from build123d import *

# Parameters (mm, degrees)
F1_DEPTH = 5


with BuildPart() as f1:
    # F0 (on Top) → F1 (new body)
    with BuildSketch(Plane.XY):
        with BuildLine():
            ThreePointArc((1.28e-08, 6), (4.9888176774, 3.3334213928), (5.5432771951, -2.2961005942))
            Line((5.5432771951, -2.2961005942), (5.5432771951, -9.5011619257))
            ThreePointArc((5.5432771951, -9.5011619257), (10.703117819, -2.5383595004), (9.2195444573, 6))
            Line((9.2195444573, 6), (1.28e-08, 6))
        make_face()
        with BuildLine():
            ThreePointArc((-5.5432771951, -2.2961005942), (-4.9888176703, 3.3334214034), (1.28e-08, 6))
            Line((1.28e-08, 6), (-9.2195444573, 6))
            ThreePointArc((-9.2195444573, 6), (-10.703117819, -2.5383595004), (-5.5432771951, -9.5011619257))
            Line((-5.5432771951, -9.5011619257), (-5.5432771951, -2.2961005942))
        make_face()
        with BuildLine():
            Line((-9.2195444573, 6), (1.28e-08, 6))
            Line((1.28e-08, 6), (9.2195444573, 6))
            ThreePointArc((9.2195444573, 6), (5.2440442409, 9.6695398029), (0, 11))
            ThreePointArc((0, 11), (-5.2440442409, 9.6695398029), (-9.2195444573, 6))
        make_face()
        with BuildLine():
            Line((-12, 6), (-9.2195444573, 6))
            ThreePointArc((-9.2195444573, 6), (-5.2440442409, 9.6695398029), (0, 11))
            Line((0, 11), (-12, 11))
            Line((-12, 11), (-12, 6))
        make_face()
        with BuildLine():
            ThreePointArc((0, 11), (5.2440442409, 9.6695398029), (9.2195444573, 6))
            Line((9.2195444573, 6), (12, 6))
            Line((12, 6), (12, 11))
            Line((12, 11), (0, 11))
        make_face()
    extrude(amount=F1_DEPTH)


solid = f1.part
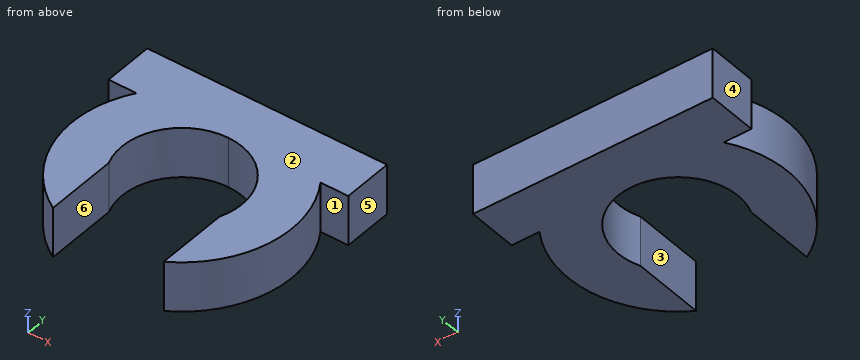
Check sheet for the modelled part. Datum: model origin and axes. Units: mm. Face numbers are marked on the shaded views. A direction names the side the tool comes from. Round coordinates to 2 decimals unless told otherwise and drop trailing zeros. Order: outer loops, then holes, each group sorted by start corner. A loop starts at its lowest first (then second) coordinate and runs counter-clockwise, first axis right, second up.
(1) Cross-section at C-C, the plane x = 9.75. Enter the section's corners in (y, z).
(2) Access from +Z, -Z, +X, -X, +Y, -Y to the whole of each face (thin tool, end or side, straight path). Record for the marked faces 1, 2 and 3.
(3) Cross-section at A-A, the plane y = 0. Enter the section's corners in (x, z).
(4) Draft check along X on the marked faces 4, 5 and 6. Enter one of: pulls with the +X half, pulls with the -X half, needs draft (parallel to the pull), parting line crosses it, or undercut.
(5) Go/stop test with flat-tipped pins: P1, Ø1.5, axis at x = -8, z = 4, coming from the -Y side; P2, Ø2, axis at x = -11, z = 3, coming from the -Y side; P3, Ø1.4, axis at x = 10, z = 2.5, coming from the -Y side; P4, Ø8, axis at x = 7, y = 1.5, coming from the -Z side. Record where each tip stops, or that it passes through.
(6) Cross-section at D-D, the plane x = 3.75. Enter the section's corners in (y, z).
(7) Scan lines: probe 1 along Y at (x, z) = (-9.5, 1.15); probe 2 along X at (y, z) = (3.5, 4.75); probe 3 along X at (y, z) = (-1.5, 4.65). Record each from-to range of solid material in increasing order.
(8) Cross-section at B-B, the plane z = 3.5. Enter the section's corners in (x, y), and give its area (3 significant figures).
Check sheet entries:
1. outline: (-5.09, 0) - (5.09, 0) - (5.09, 5) - (-5.09, 5) - close; (6, 0) - (11, 0) - (11, 5) - (6, 5) - close
2. face 1: +Z, -Z, +X
2. face 2: +Z, +X, -X, +Y, -Y
2. face 3: +Z, -Z, -Y
3. outline: (-11, 0) - (-6, 0) - (-6, 5) - (-11, 5) - close; (6, 0) - (11, 0) - (11, 5) - (6, 5) - close
4. face 4: pulls with the -X half
4. face 5: pulls with the +X half
4. face 6: undercut
5. P1: stops at y = -8.27
5. P2: stops at y = -4.58
5. P3: stops at y = -5.87
5. P4: stops at z = 0
6. outline: (4.68, 0) - (11, 0) - (11, 5) - (4.68, 5) - close
7. probe 1: y = -5.55 to 5.55, 6 to 11
7. probe 2: x = -10.43 to -4.87, 4.87 to 10.43
7. probe 3: x = -10.9 to -5.81, 5.81 to 10.9
8. outline: (-12, 6) - (-9.22, 6) arc R11 ccw to (-5.54, -9.5) - (-5.54, -2.3) arc R6 cw (long way) to (5.54, -2.3) - (5.54, -9.5) arc R11 ccw to (9.22, 6) - (12, 6) - (12, 11) - (-12, 11) - close
8. area: 261 mm2
